Read the model definition and answer for the solid it produces. Units are mm, in the model's axes. A direction names the side the tool comes from. Give positions to 0.01 mm unless a question says otherwise; leave off trailing zeros. Order: outer loops, then holes, each group sorted by start corner. A loop starts at its lowest first (then second) coordinate and runs counter-clockwise, first axis right, second up. Notation, with made-up numbers: (29.25, 7) -> (35.25, 7) arc R19 cw to (35.25, 25) -> close; hole circle Ø2 at (4.25, -4). An arc over 180 degrees is marked (long way). Answer as CSV lines item,"result". Start each with the question number.
1) The mould has two halves that part along X. Classify faces 1 (the face through (17, 14, 12)), 2 (the face through (15, 0, 30)), 3 (the face through (-29.5, -11, 10)): +X half, -X half, draft (parallel to the pull), parting line (faces both ways), or undercut.
2) For faces 4 (the face through (11.527, -0.21, 22.574)), 5 (the face through (17, 8, 3)), 6 (the face through (-27.5, 0, 5)), 7 (the face through (3.93, -13.5, 24.06)), 8 (the face through (1, 0.14, 16.43)), determine the directions among +Z, -Z, +X, -X, +Y, -Y from which every point of the face is accessible in a straight line to the end or side of a thin tool.
3) Find section A-A (x = 17.5). Determine the outline of the cut face in (y, z).
4) Find section C-C (z = 22). Determine the outline of the cut face in (x, y).
5) Straight lines are drawn through the part: L1, parallel to Z at x = 17, y = 0; L2, parallel to X at y = 13, z = 5.25; L3, parallel to X at y = 11.5, z = 2.75. For each, find the intervals that lie inside material, in ascending order. Write a range as from..to.
6) Find section B-B (y = -4). State how many separate pieces and enclosed holes the cut face has, and give its area (3 significant figures).
7) Find section D-D (x = 23.5). Determine the outline of the cut face in (y, z).
8) Flat-ended cylindrical pins translate along their axes: pin 1 Ø4 at (x, z) = (-18, 3) entering from +Y; pin 2 Ø1.5 at (y, z) = (-3, 21.5) entering from -X; pin 3 Ø5 at (x, z) = (-22.5, 19.5) entering from -Y. Find the tip coordinate at first contact, or state that the pin passes through.
```python
from build123d import *

# Parameters (mm, degrees)
F0_W      = 55
F0_H      = 30
F1_DEPTH  = 30
F2_W      = 30
F2_H      = 15
F3_DEPTH  = 30.001
F5_DEPTH  = 7
F6_F1_R   = 5
F6_F2_R   = 5
F7_SIZE   = 2
F9_DEPTH  = 30.001
F10_R     = 5
F12_DEPTH = 2
F13_R     = 3
F14_DEPTH = 15
F15_R     = 5
F15_R_2   = 3
F16_DEPTH = 4
F17_SIZE  = 1.99999


# Not quite as in the source:
# - a fillet or chamfer is up to 0.001 mm smaller than in the source, because OpenCascade refuses the exact size
# - a pattern or mirror of a feature is missing from the dataset's text; its kind, count and spacing are read off the source's solid


with BuildPart() as f1:
    # F0 (on Top) → F1 (new body)
    with BuildSketch(Plane.XY):
        Rectangle(F0_W, F0_H)
    extrude(amount=F1_DEPTH)

    # F2 (on face) → F3 (cut, through all)
    with BuildSketch(Plane.XZ.offset(15)):
        with Locations((-12.5, 22.5)):
            Rectangle(F2_W, F2_H)
    extrude(amount=-F3_DEPTH, mode=Mode.SUBTRACT)

    # F4 (on face) → F5 (cut)
    with BuildSketch(Plane.XZ.offset(15)):
        with BuildLine():
            Line((-25, 0), (-10, 0))
            ThreePointArc((-10, 0), (-17.5, 7.5), (-25, 0))
        make_face()
        with BuildLine():
            ThreePointArc((25, 0), (17.5, 7.5), (10, 0))
            Line((10, 0), (25, 0))
        make_face()
    f5 = extrude(amount=-F5_DEPTH, mode=Mode.SUBTRACT)

    # F5_copies: F5 across plane
    add(f5.mirror(Plane.ZX), mode=Mode.SUBTRACT)

    # F6: fillet of radius 5 on 4 edges, made by hand

    # F6_f1
    f6_f1_edges = [f1.edges().sort_by_distance(p)[0] for p in [
        (2.5, 0, 15),
    ]]
    fillet(f6_f1_edges, radius=F6_F1_R)

    # F6_f2
    f6_f2_edges = [f1.edges().sort_by_distance(p)[0] for p in [
        (-15, -15, 15),
        (-15, 15, 15),
        (-27.5, 0, 15),
        (1.0355339059, 15, 16.4644660941),
        (1.0355339059, -15, 16.4644660941),
    ]]
    fillet(f6_f2_edges, radius=F6_F2_R)

    # F7
    f7_edges = [f1.edges().sort_by_distance(p)[0] for p in [
        (17.5, -15, 30),
        (3.964466, -13.535534, 30),
        (27.5, 0, 30),
        (2.5, 0, 30),
        (17.5, 15, 30),
        (3.964466, 13.535534, 30),
    ]]
    chamfer(f7_edges, length=F7_SIZE)

    # F8 (on face) → F9 (cut, through all)
    with BuildSketch(Plane.XZ.offset(15)):
        with BuildLine():
            Line((20.0235929713, 24), (15.0235929713, 24))
            ThreePointArc((15.0235929713, 24), (11.4880590653, 22.5355339059), (10.0235929713, 19))
            Line((10.0235929713, 19), (10.0235929713, 14))
            Line((10.0235929713, 14), (25.0235929713, 14))
            Line((25.0235929713, 14), (25.0235929713, 19))
            ThreePointArc((25.0235929713, 19), (23.5591268772, 22.5355339059), (20.0235929713, 24))
        make_face()
    extrude(amount=-F9_DEPTH, mode=Mode.SUBTRACT)

    # F10
    f10_edges = [f1.edges().sort_by_distance(p)[0] for p in [
        (17.523593, -15, 14),
        (17.523593, 15, 14),
    ]]
    fillet(f10_edges, radius=F10_R)

    # F11 (on face) → F12 (join)
    with BuildSketch(Plane(origin=(-27.5, 0, 0), x_dir=(0, -1, 0), z_dir=(-1, 0, 0))):
        with BuildLine():
            Line((-14, 10), (-8, 10))
            ThreePointArc((-8, 10), (-11, 13), (-14, 10))
        make_face()
        with BuildLine():
            ThreePointArc((-14, 10), (-11, 7), (-8, 10))
            Line((-8, 10), (-14, 10))
        make_face()
        with BuildLine():
            Line((14, 10), (8, 10))
            ThreePointArc((8, 10), (11, 7), (14, 10))
        make_face()
        with BuildLine():
            ThreePointArc((14, 10), (11, 13), (8, 10))
            Line((8, 10), (14, 10))
        make_face()
    extrude(amount=F12_DEPTH)

    # F13 (on face) → F14 (join)
    with BuildSketch(Plane.XY.offset(15)):
        with Locations((-17.5, 0)):
            Circle(F13_R)
    extrude(amount=F14_DEPTH)

    # F15 (on face) → F16 (join)
    with BuildSketch(Plane.XY.offset(30)):
        with Locations((-17.5, 0)):
            Circle(F15_R)
        with Locations((-17.5, 0)):
            Circle(F15_R_2, mode=Mode.SUBTRACT)
    extrude(amount=-F16_DEPTH)

    # F17 (size 2 in the source; OpenCascade refuses exactly that, so slightly less here)
    f17_edges = [f1.edges().sort_by_distance(p)[0] for p in [
        (-22.5, 0, 26),
    ]]
    chamfer(f17_edges, length=F17_SIZE)


solid = f1.part
```
Findings below:
1,face 1,"undercut"
1,face 2,"draft"
1,face 3,"-X half"
2,face 4,"+Y, -Y"
2,face 5,"-Z, +Y"
2,face 6,"-Z, -X"
2,face 7,"+Z, -X, -Y"
2,face 8,"+Z, +Y, -Y"
3,outline,"(-15, 7.5) -> (-8, 7.5) -> (-8, 0) -> (8, 0) -> (8, 7.5) -> (15, 7.5) -> (15, 9) arc R5 ccw to (10, 14) -> (-10, 14) arc R5 ccw to (-15, 9) -> close; (-15, 24) -> (15, 24) -> (15, 28) -> (13, 30) -> (-13, 30) -> (-15, 28) -> close"
4,outline,"circle Ø6 at (-17.5, 0); (2.5, -10) arc R5 ccw to (7.5, -15) -> (11.02, -15) -> (11.02, 15) -> (7.5, 15) arc R5 ccw to (2.5, 10) -> close; (24.02, -15) -> (27.5, -15) -> (27.5, 15) -> (24.02, 15) -> close"
5,L1,"0..14, 24..30"
5,L2,"-27.5..-22.86, -12.14..12.14, 22.86..27.5"
5,L3,"-27.5..-24.48, -10.52..10.52, 24.48..27.5"
6,separate pieces,"2"
6,enclosed holes,"1"
6,area,"1,070 mm²"
7,outline,"(-15, 4.5) -> (-8, 4.5) -> (-8, 0) -> (8, 0) -> (8, 4.5) -> (15, 4.5) -> (15, 9) arc R5 ccw to (10, 14) -> (-10, 14) arc R5 ccw to (-15, 9) -> close; (-15, 22.59) -> (15, 22.59) -> (15, 28) -> (13, 30) -> (-13, 30) -> (-15, 28) -> close"
8,pin 1,"y = 8"
8,pin 2,"x = -19.48"
8,pin 3,"y = -1.66"
